Drawing for the job (mm, zero at the part's lowest x, y, z). A direction names the side the tool comes from. Round coordinates to 2 decimals unless told otherwise and drop trailing zeros. Order: outer loops, then holes, each group sorted by start corner. A loop starts at its lowest first (then second) coordinate and runs counter-clockwise, first axis right, second up. Notation, with made-up numbers: (42.25, 70.25) - (100.25, 70.25) arc R25 cw to (100.25, 109.25) - close; hole circle Ø1 at (70, 2). An arc over 180 degrees is marked (long way). Answer as a JSON object with one key per item and string values.
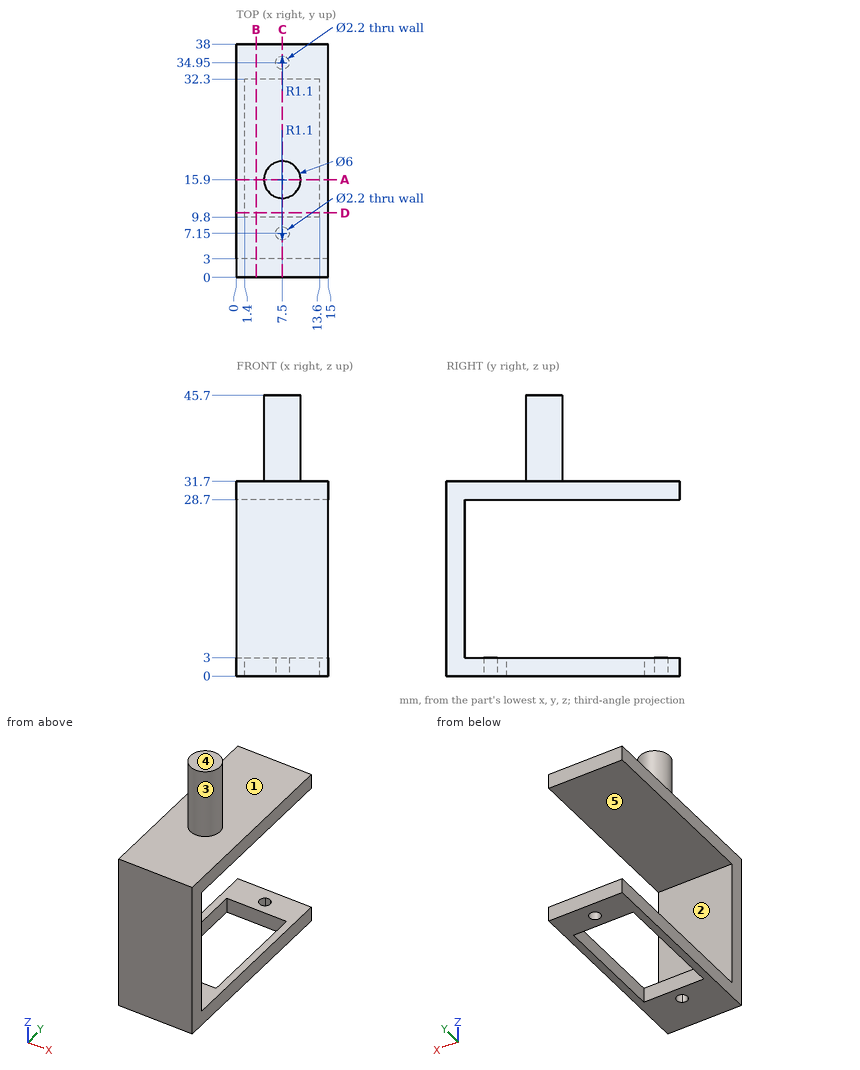
Item 1: Probe L1, parallel to Y at x = 7.5, z = 1.4; L2, parallel to X at y = 34.95, z = 0.9; L3, parallel to Z at x = 2.75, y = 34.5. List the from-to ranges inside material, lowest first. Write a range as from..to.
Taken from the geometry:
{"L1": "0..6.05, 8.25..9.8, 32.3..33.85, 36.05..38", "L2": "0..6.4, 8.6..15", "L3": "0..3, 28.7..31.7"}
Item 2: Cut at C-C (x = 7.5). Write the cut outline in (y, z).
Taken from the geometry:
{"outline": "(0, 0) - (6.05, 0) - (6.05, 3) - (3, 3) - (3, 28.7) - (38, 28.7) - (38, 31.7) - (18.9, 31.7) - (18.9, 45.7) - (12.9, 45.7) - (12.9, 31.7) - (0, 31.7) - close; (8.25, 0) - (9.8, 0) - (9.8, 3) - (8.25, 3) - close; (32.3, 0) - (33.85, 0) - (33.85, 3) - (32.3, 3) - close; (36.05, 0) - (38, 0) - (38, 3) - (36.05, 3) - close"}
Item 3: Two-plate mould, pull along Z, no slides. Class the marked faces 1, 2 and 3: pulls with the +Z half, pulls with the -Z half, needs draft (parallel to the pull), parting line crosses it, or undercut.
Taken from the geometry:
{"face 1": "pulls with the +Z half", "face 2": "undercut", "face 3": "needs draft"}
Item 4: Tool access for the marked faces 4 and 5: list every direction of +Z, -Z, +X, -X, +Y, -Y with a clear straight run to the whole face (end or side of a thin tool).
Taken from the geometry:
{"face 4": "+Z, +X, -X, +Y, -Y", "face 5": "+X, -X, +Y"}
Item 5: Cut at D-D (y = 10.5). Write the cut outline in (x, z).
Taken from the geometry:
{"outline": "(0, 0) - (1.4, 0) - (1.4, 3) - (0, 3) - close; (0, 28.7) - (15, 28.7) - (15, 31.7) - (0, 31.7) - close; (13.6, 0) - (15, 0) - (15, 3) - (13.6, 3) - close"}
Item 6: Drop flat-ended pins along their axis: P1, Ø4.5, axis at x = 5.5, z = 21, coming from the +Y side; P2, Ø7.5, axis at x = 6, y = 18, coming from the -Z side. Give the stop position or say it passes through.
Taken from the geometry:
{"P1": "y = 3", "P2": "z = 28.7"}
Item 7: Cut at B-B (x = 3.25). Write the cut outline in (y, z).
Taken from the geometry:
{"outline": "(0, 0) - (9.8, 0) - (9.8, 3) - (3, 3) - (3, 28.7) - (38, 28.7) - (38, 31.7) - (0, 31.7) - close; (32.3, 0) - (38, 0) - (38, 3) - (32.3, 3) - close"}
Item 8: Cut at A-A (y = 15.9). Write the cut outline in (x, z), plus the area to 3 significant figures.
Taken from the geometry:
{"outline": "(0, 0) - (1.4, 0) - (1.4, 3) - (0, 3) - close; (0, 28.7) - (15, 28.7) - (15, 31.7) - (10.5, 31.7) - (10.5, 45.7) - (4.5, 45.7) - (4.5, 31.7) - (0, 31.7) - close; (13.6, 0) - (15, 0) - (15, 3) - (13.6, 3) - close", "area": "137 mm2"}
